Study the drawing (mm; zero at the part's minimum x, y, z) and answer. A direction names the side the tool comes from. Give positions to 0.01 mm unless a question says otherwise; leave off trailing zeros. Order: outer loops, then holes, each group sorted by start corner. A loop starts at its lowest first (then second) coordinate and runs counter-clockwise, first axis right, second up. Notation, with made-up numbers: (73.25, -21.75) - (128.25, -21.75) arc R35 ccw to (128.25, 10.25) - close; hole circle Ø7 at (61, 4). An arc over 180 degrees is marked (long way). Put each result on its own line as item: value.
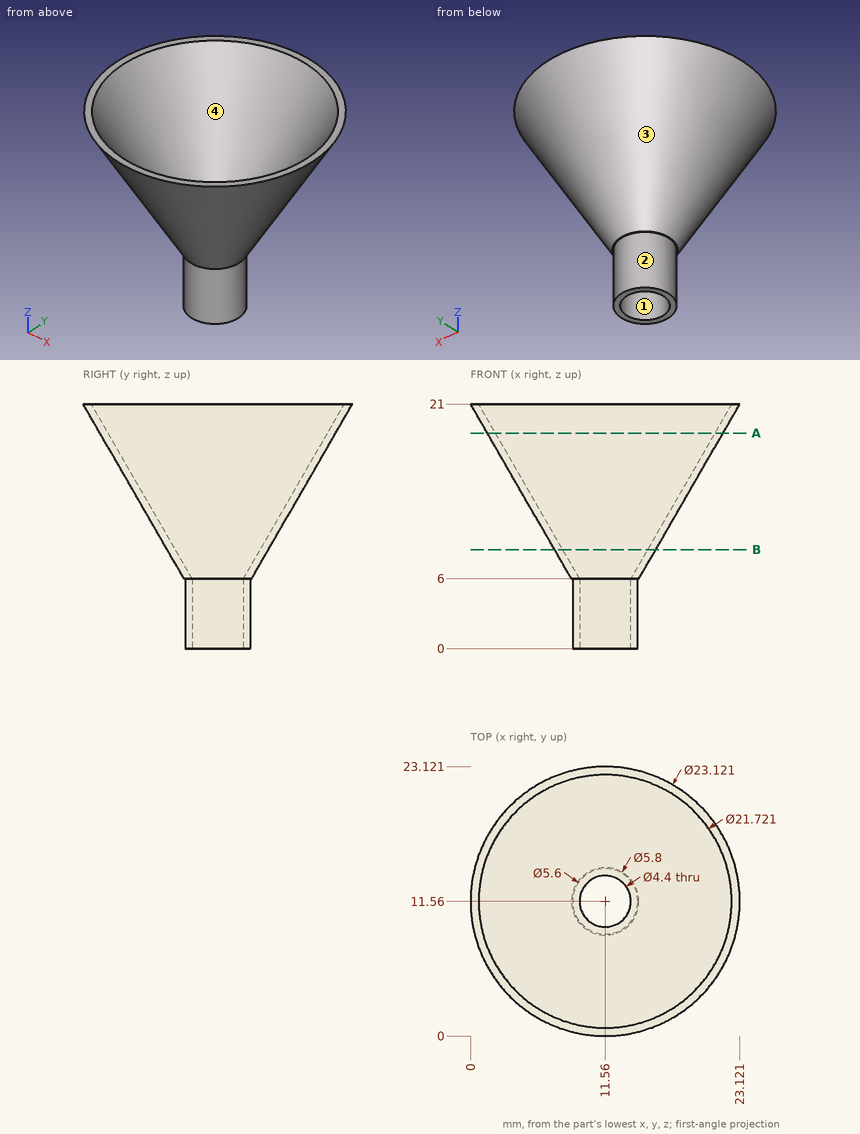
(1) Straight lines are drawn through the part: line 1 (Y direction, x = 11.5, z = 11) (1 decimal); line 2 (Y direction, x = 7.75, z = 13.75) (1 decimal). For each, find the intervals that lie inside material, in ascending order.
Geometry check:
line 1: y = 5.8 to 6.5, 16.6 to 17.3
line 2: y = 5.2 to 6.1, 17 to 17.9
(2) Section B-B, the plane z = 8.5 is taken. Write down the section's boundary in (x, y).
Geometry check:
outline: circle Ø8.69 at (11.56, 11.56); hole circle Ø7.29 at (11.56, 11.56)
(3) Given pin 1 (1 mm diameter, centred on x = 7.5, y = 13.5, fed in from +Z); pin 2 (3 mm diameter, centred on y = 12.5, z = 15, fed in from +X) (1 decimal); pin 3 (10 mm diameter, centred on y = 5, z = 8, fed in from +X), each flat-ended and moving along its own axis, determine where each tip first touches the part or whether it passes through.
Geometry check:
pin 1: stops at z = 10.85
pin 2: stops at x = 20.5
pin 3: stops at x = 16.86
(4) A tool of negligible diameter and unlimited length cuts with its end or side. For the marked faces 1 and 2, from which of +Z, -Z, +X, -X, +Y, -Y can it reach the whole face along a straight path? Write none if from no direction.
Geometry check:
face 1: +Z, -Z
face 2: -Z
(5) Determine the mould class of the marked faces 3 and 4 for opening direction X: pulls with the +X half, pulls with the -X half, needs draft (parallel to the pull), parting line crosses it, or undercut.
Geometry check:
face 3: parting line crosses it
face 4: undercut
(6) Section A-A, the plane z = 18.5 is taken. Write down the section's boundary in (x, y).
Geometry check:
outline: circle Ø20.23 at (11.56, 11.56); hole circle Ø18.83 at (11.56, 11.56)
